```python
from build123d import *

# Parameters (mm, degrees)
CROQUIS1_R              = 63.75
SALIENTE_EXTRUIR1_DEPTH = 29.32
CROQUIS2_R              = 31.625
CORTAR_EXTRUIR1_DEPTH   = 2
REDONDEO2_R             = 4
REDONDEO3_R             = 14
CROQUIS4_R              = 31.625
CORTAR_EXTRUIR3_DEPTH   = 2
CROQUIS5_R              = 27.12
CORTAR_EXTRUIR4_DEPTH   = 2
REDONDEO4_R             = 14
CROQUIS6_R              = 4.05
CORTAR_EXTRUIR5_DEPTH   = 30
REDONDEO5_R             = 2
REDONDEO6_R             = 2


# Some blends are built 0.0001 mm under size
with BuildPart() as part:
    # Croquis1 → Saliente-Extruir1 (new, symmetric)
    with BuildSketch(Plane.XY):
        with Locations(Location((0, 0, 0), (0, 0, 180))):
            Circle(CROQUIS1_R)
    extrude(amount=SALIENTE_EXTRUIR1_DEPTH, both=True)

    # Croquis2 → Cortar-Extruir1 (cut)
    with BuildSketch(Plane.XY.offset(29.32)):
        Circle(CROQUIS2_R)
    extrude(amount=-CORTAR_EXTRUIR1_DEPTH, mode=Mode.SUBTRACT)

    # Redondeo2
    # the kernel refuses this fillet: 4 mm, written as the material it adds along each edge
    with BuildSketch(Plane(origin=(0, 0, 27.32), x_dir=(1, 0, 0), z_dir=(0, -1, 0))) as redondeo2_piece_1:
        with BuildLine():
            CenterArc((28.160898385, 4), REDONDEO2_R, 270, 60)
            Line((28.160898385, 0), (28.160898385, -0.08))
            Line((28.160898385, -0.08), (31.625, -0.08))
            Line((31.625, -0.08), (31.705, 0))
            ThreePointArc((31.705, 0), (31.705, 1), (31.694282032, 1.96))
            Line((31.694282032, 1.96), (31.625, 2))
        make_face()
    revolve(axis=Axis((0, 0, 27.32), (0, 0, 1)))

    # Redondeo3
    redondeo3_edges = [part.edges().sort_by_distance(p)[0] for p in [
        (63.75, 0, 29.32),
    ]]
    fillet(redondeo3_edges, radius=REDONDEO3_R)

    # Croquis4 → Cortar-Extruir3 (cut)
    with BuildSketch(Plane(origin=(0, 0, -29.32), x_dir=(-1, 0, 0), z_dir=(0, 0, -1))):
        Circle(CROQUIS4_R)
    extrude(amount=-CORTAR_EXTRUIR3_DEPTH, mode=Mode.SUBTRACT)

    # Croquis5 → Cortar-Extruir4 (cut)
    with BuildSketch(Plane(origin=(0, 0, -27.32), x_dir=(-1, 0, 0), z_dir=(0, 0, -1))):
        Circle(CROQUIS5_R)
    extrude(amount=-CORTAR_EXTRUIR4_DEPTH, mode=Mode.SUBTRACT)

    # Redondeo4
    redondeo4_edges = [part.edges().sort_by_distance(p)[0] for p in [
        (63.75, 0, -29.32),
    ]]
    fillet(redondeo4_edges, radius=REDONDEO4_R)

    # Croquis6 → Cortar-Extruir5 (cut)
    with BuildSketch(Plane(origin=(0, 0, -25.32), x_dir=(-1, 0, 0), z_dir=(0, 0, -1))):
        Circle(CROQUIS6_R)
    extrude(amount=-CORTAR_EXTRUIR5_DEPTH, mode=Mode.SUBTRACT)

    # Redondeo5
    redondeo5_edges = [part.edges().sort_by_distance(p)[0] for p in [
        (27.12, 0, -27.32),
    ]]
    fillet(redondeo5_edges, radius=REDONDEO5_R - 0.0001)  # a hair under: the kernel refuses the full size

    # Redondeo6
    redondeo6_edges = [part.edges().sort_by_distance(p)[0] for p in [
        (31.625, 0, -27.32),
    ]]
    fillet(redondeo6_edges, radius=REDONDEO6_R - 0.0001)  # a hair under: the kernel refuses the full size


solid = part.part
```
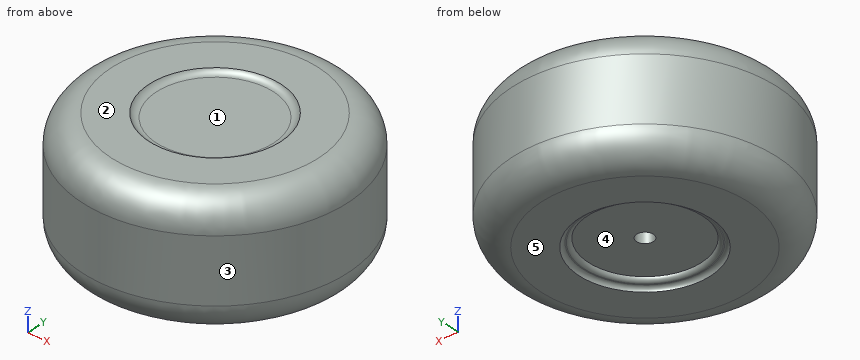
Part model, mm, in its own coordinate system. Face numbers are marked on the shaded views. A direction names the side the tool comes from. Coordinates: 2 decimals unless noted, no trailing zeros. Loops run counter-clockwise (first coordinate to the right, second up) from the corner with the lowest first, then second, coordinate; pieces in that order, holes last. Notation, with made-up numbers: (21, -26.75) - (63, -26.75) arc R18 cw to (63, -18.75) - close; hole circle Ø4 at (6, 28). An arc over 180 degrees is marked (long way). Write item = value, one per line. Start each with the question number.
Item 1: Mould opens along Y. For the marked faces 3, 4 and 5 say: released by +Y, released by -Y, zero draft, split by the parting line, or undercut.
Item 2: Cut at C-C, the plane z = -13. Give the cut face in (x, y).
Item 3: 3-axis set-ups, long thin cutter, end or side, ignore diameter. For the marked faces 1 and 2: which of +Z, -Z, +X, -X, +Y, -Y reach the whole face in a straight line?
Item 4: Wall check: L1, parallel to Y at x = 0, z = -16; L2, parallel to Z at x = -1.5, y = 19; L3, parallel to X at y = 0.5, z = -25. Give the ranges that are in metal, low to high. Write a range as from..to.
Item 5: Cut at D-D, the plane z = 6.5. Give the cut face in (x, y), and give its area (3 significant figures).
Item 6: Flat gauge pins, fed straight in: pin 1 Ø3 at (x, z) = (23.5, 18.5) entering from +Y; pin 2 Ø9 at (x, y) = (-1, 1) entering from -Z; pin 3 Ø10 at (y, z) = (39.5, -8.5) entering from -X. Where does each tip first touch, or does it go through?
The answers:
q1.face_3 = split by the parting line
q1.face_4 = undercut
q1.face_5 = zero draft
q2.outline = circle Ø127.5 at (0, 0); hole circle Ø8.1 at (0, 0)
q3.face_1 = +Z
q3.face_2 = +Z, +X, -X, +Y, -Y
q4.L1 = -63.73..-4.05, 4.05..63.73
q4.L2 = -25.32..27.32
q4.L3 = -59.86..-4.02, 4.02..59.86
q5.outline = circle Ø127.5 at (0, 0)
q5.area = 12,800 mm2
q6.pin_1 = 59.53
q6.pin_2 = -25.32
q6.pin_3 = -53.61
